from build123d import *

# Parameters (mm, degrees)
CROQUIS1_R              = 110
SALIENTE_EXTRUIR1_DEPTH = 10
CORTAR_EXTRUIR1_DEPTH   = 10
CROQUIS4_R              = 2
CORTAR_EXTRUIR3_DEPTH   = 156.884572681
CROQUIS5_R              = 2.45
CROQUIS5_R_2            = 2.25
CORTAR_EXTRUIR4_DEPTH   = 7
CROQUIS8_R              = 5
CORTAR_EXTRUIR5_DEPTH   = 156.884572681
CROQUIS11_R             = 2.5
CORTAR_EXTRUIR6_DEPTH   = 10
CROQUIS12_R             = 1.5
CORTAR_EXTRUIR7_DEPTH   = 10
CORTAR_EXTRUIR8_DEPTH   = 156.884572681
CROQUIS14_R             = 2.5
CORTAR_EXTRUIR9_DEPTH   = 5
CROQUIS17_R             = 2.186456698
CORTAR_EXTRUIR10_DEPTH  = 156.884572681


with BuildPart() as part:
    # Croquis1 → Saliente-Extruir1 (new body)
    with BuildSketch(Plane(origin=(0, 0, 0), x_dir=(1, 0, 0), z_dir=(0, 1, 0))):
        with Locations(Location((0, 0, 0), (0, 0, 270))):
            Circle(CROQUIS1_R)
    extrude(amount=SALIENTE_EXTRUIR1_DEPTH)

    # Croquis2 → Cortar-Extruir1 (cut)
    with BuildSketch(Plane(origin=(0, 10, 0), x_dir=(1, 0, 0), z_dir=(0, 1, 0))):
        with BuildLine():
            Line((-40.925729633, -32.159166383), (-7.30856573, -37.247023602))
            ThreePointArc((-7.30856573, -37.247023602), (-5.504506631, -39.694546997), (-7.952030025, -41.498606096))
            Line((-7.952030025, -41.498606096), (-41.569193929, -36.410748877))
            ThreePointArc((-41.569193929, -36.410748877), (-43.373253028, -33.963225482), (-40.925729633, -32.159166383))
        make_face()
        with BuildLine():
            Line((-11.802959176, -66.941742857), (-45.419686894, -61.851004448))
            ThreePointArc((-45.419686894, -61.851004448), (-47.223536218, -59.403326443), (-44.775858213, -57.599477119))
            Line((-44.775858213, -57.599477119), (-11.159130495, -62.690215528))
            ThreePointArc((-11.159130495, -62.690215528), (-9.355281171, -65.137893533), (-11.802959176, -66.941742857))
        make_face()
    extrude(amount=-CORTAR_EXTRUIR1_DEPTH, mode=Mode.SUBTRACT)

    # Croquis4 → Cortar-Extruir3 (cut, through all)
    with BuildSketch(Plane.XZ):
        with Locations(Location((-6.850793921, -14.673517402, 0), (0, 0, 270))):
            Circle(CROQUIS4_R)
        with Locations(Location((14.673517402, -6.850793921, 0), (0, 0, 270))):
            Circle(CROQUIS4_R)
        with Locations(Location((-14.673517402, 6.850793921, 0), (0, 0, 270))):
            Circle(CROQUIS4_R)
        with Locations(Location((6.850793921, 14.673517402, 0), (0, 0, 270))):
            Circle(CROQUIS4_R)
    extrude(amount=-CORTAR_EXTRUIR3_DEPTH, mode=Mode.SUBTRACT)

    # Croquis5 → Cortar-Extruir4 (cut)
    with BuildSketch(Plane(origin=(0, 10, 0), x_dir=(1, 0, 0), z_dir=(0, 1, 0))):
        with Locations(Location((-48.761952302, 28.58020577, 0), (0, 0, 270))):
            Circle(CROQUIS5_R)
        with Locations(Location((-55.046952396, -12.946879052, 0), (0, 0, 270))):
            Circle(CROQUIS5_R)
        with Locations(Location((63.492012818, 11.590903863, 0), (0, 0, 270))):
            Circle(CROQUIS5_R)
        with Locations(Location((57.207012724, -29.936180959, 0), (0, 0, 270))):
            Circle(CROQUIS5_R)
        with Locations(Location((85.994568937, 8.185209293, 0), (0, 0, 270))):
            Circle(CROQUIS5_R_2)
        with Locations(Location((79.709568842, -33.341875529, 0), (0, 0, 270))):
            Circle(CROQUIS5_R_2)
    extrude(amount=-CORTAR_EXTRUIR4_DEPTH, mode=Mode.SUBTRACT)

    # Croquis8 → Cortar-Extruir5 (cut, through all)
    with BuildSketch(Plane(origin=(0, 10, 0), x_dir=(1, 0, 0), z_dir=(0, 1, 0))):
        with Locations(Location((0, 0, 0), (0, 0, 270))):
            Circle(CROQUIS8_R)
    extrude(amount=-CORTAR_EXTRUIR5_DEPTH, mode=Mode.SUBTRACT)

    # Croquis11 → Cortar-Extruir6 (cut)
    with BuildSketch(Plane.XZ):
        with Locations(Location((-83.094178071, -12.302746472, 0), (0, 0, 270))):
            Circle(CROQUIS11_R)
        with Locations(Location((12.302746472, -83.094178071, 0), (0, 0, 270))):
            Circle(CROQUIS11_R)
        with Locations(Location((83.094178071, 12.302746472, 0), (0, 0, 270))):
            Circle(CROQUIS11_R)
        with Locations(Location((-12.302746472, 83.094178071, 0), (0, 0, 270))):
            Circle(CROQUIS11_R)
    extrude(amount=-CORTAR_EXTRUIR6_DEPTH, mode=Mode.SUBTRACT)

    # Croquis12 → Cortar-Extruir7 (cut)
    with BuildSketch(Plane(origin=(0, 10, 0), x_dir=(1, 0, 0), z_dir=(0, 1, 0))):
        with Locations(Location((34.860845045, 39.241411656, 0), (0, 0, 270))):
            Circle(CROQUIS12_R)
        with Locations(Location((45.170870311, 92.869347277, 0), (0, 0, 270))):
            Circle(CROQUIS12_R)
        with Locations(Location((-12.198549191, 103.898676632, 0), (0, 0, 270))):
            Circle(CROQUIS12_R)
        with Locations(Location((-22.508574457, 50.270741011, 0), (0, 0, 270))):
            Circle(CROQUIS12_R)
    extrude(amount=-CORTAR_EXTRUIR7_DEPTH, mode=Mode.SUBTRACT)

    # Croquis13 → Cortar-Extruir8 (cut, through all)
    with BuildSketch(Plane(origin=(0, 10, 0), x_dir=(1, 0, 0), z_dir=(0, 1, 0))):
        Polygon((-39.036973786, -3.44597737), (-30.835647873, -4.687223519), (-28.104551712, 13.358036658), (-36.305877626, 14.599282808), align=None)
    extrude(amount=-CORTAR_EXTRUIR8_DEPTH, mode=Mode.SUBTRACT)

    # Croquis14 → Cortar-Extruir9 (cut)
    with BuildSketch(Plane(origin=(0, 10, 0), x_dir=(1, 0, 0), z_dir=(0, 1, 0))):
        with Locations(Location((-61.128340654, 82.810846507, 0), (0, 0, 270))):
            Circle(CROQUIS14_R)
        with Locations(Location((-82.810846507, -61.128340654, 0), (0, 0, 270))):
            Circle(CROQUIS14_R)
        with Locations(Location((61.128340654, -82.810846507, 0), (0, 0, 270))):
            Circle(CROQUIS14_R)
        with Locations(Location((82.810846507, 61.128340654, 0), (0, 0, 270))):
            Circle(CROQUIS14_R)
    extrude(amount=-CORTAR_EXTRUIR9_DEPTH, mode=Mode.SUBTRACT)

    # Croquis17 → Cortar-Extruir10 (cut, through all)
    with BuildSketch(Plane.XZ):
        with Locations(Location((-28.290947151, 16.202590632, 0), (0, 0, 270))):
            Circle(CROQUIS17_R)
        with Locations(Location((16.202590632, 28.290947151, 0), (0, 0, 270))):
            Circle(CROQUIS17_R)
        with Locations(Location((28.290947151, -16.202590632, 0), (0, 0, 270))):
            Circle(CROQUIS17_R)
        with Locations(Location((-16.202590632, -28.290947151, 0), (0, 0, 270))):
            Circle(CROQUIS17_R)
    extrude(amount=-CORTAR_EXTRUIR10_DEPTH, mode=Mode.SUBTRACT)


solid = part.part
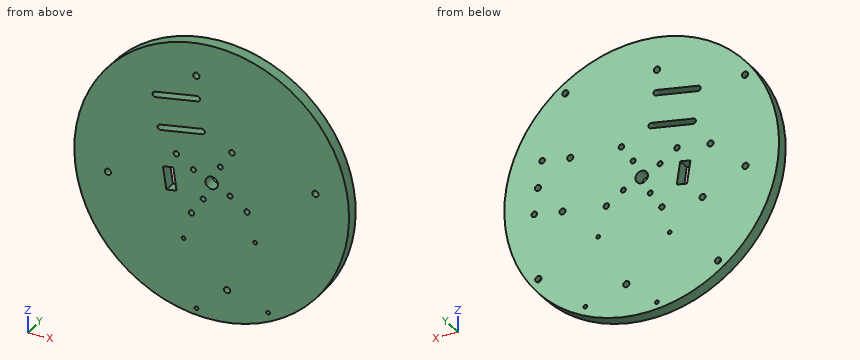
Input: part model. Units: mm. Frame: model coordinates. Give positions to 0.01 mm unless a question says otherwise; leave off trailing zeros. Loops run counter-clockwise (first coordinate to the right, second up) from the corner with the lowest first, then second, coordinate; pieces in that order, holes last. Notation, with made-up numbers: M -32.5,-22 L -6.5,-22 A29 cw -6.5,11 Z; hole C 68.5,44 d7. An arc over 180 degrees is marked long. Use one line per item in the form item = value.
1. Line query: L1, parallel to X at y = 5.25, z = 83.5; L2, parallel to X at y = 5.5, z = 30; L3, parallel to Z at x = -43, y = 2.75. Output: solid intervals per line, ascending.
Numbers:
L1 = -71.61 to -14.77, -9.84 to 58.73, 63.53 to 71.61
L2 = -105.83 to 14.84, 17.57 to 54.76, 59.66 to 105.83
L3 = -101.25 to 33.04, 35.53 to 57.87, 62.22 to 101.25
2. Section query B-B, the plane z = 0. Return the cut outline in (x, y).
Numbers:
outline = M -110,0 L -38.52,0 L -38.52,10 L -110,10 Z; M -30.13,0 L -5,0 L -5,10 L -30.13,10 Z; M 5,0 L 110,0 L 110,10 L 5,10 Z
3. Section query A-A, the plane x = 0. Return the cut outline in (y, z), and give its area (3 significant figures).
Numbers:
outline = M 0,-110 L 10,-110 L 10,-5 L 0,-5 Z; M 0,5 L 10,5 L 10,110 L 0,110 Z
area = 2,100 mm²
4. First-contact query: pin 1 (5 mm diameter, centred on x = -23, y = 1, fed in from +Z); pin 2 (2 mm diameter, centred on y = 3.5, z = 49.5, fed in from -X); pin 3 (3 mm diameter, centred on x = -6.85, z = -14.67, fed in from +Y); pin 4 (1 mm diameter, centred on y = 6, z = -37, fed in from -X). Flat tips, straight axial feed; report the tip coordinate or a pass-through.
Numbers:
pin_1 = 108.07
pin_2 = -98.73
pin_3 = through
pin_4 = -103.77
